Autodesk Inventor part; units mm, degrees
ref_plane "YZ Plane" through (0, 0, 0) normal (1, 0, 0) x (0, 1, 0)
ref_plane "XZ Plane" through (0, 0, 0) normal (0, 1, 0) x (-1, 0, 0)
ref_plane "XY Plane" through (0, 0, 0) normal (0, 0, 1) x (1, 0, 0)
sketch "Szkic1" plane through (0, 0, 0) normal (0, 0, 1) x (1, 0, 0)
  circle A0 centre (0, 0) radius 3
  circle A1 centre (0, 0) radius 6
  point P0 (0, 0)
  dimension "d0" = 12
extrude "Wyciągnięcie proste1" add sketch "Szkic1" against normal blind 1 contours A0 | A1
sketch "Szkic2" plane through (0, 0, 0) normal (0, 0, 1) x (1, 0, 0)
  circle A0 centre (0, 0) radius 6
  circle A1 centre (0, 0) radius 5
  point P0 (0, 0)
  dimension "d3" = 1
extrude "Wyciągnięcie proste2" add sketch "Szkic2" along normal blind 10
full round fillet "Zaokrąglenie1" first side at (4.9353, -0.8021, 6.6667) centre faces at (5.6086, -0.4786, 10) second side at (5.9223, -0.9625, 2.6667)
sketch "Szkic3" plane through (0, 0, 0) normal (0, 1, 0) x (-1, 0, 0)
  line L0 (-6, -1) -> (6, -1)
  line L1 (6, 9.5) -> (-6, 9.5)
  line L2 (0, 3) -> (25, 3)
  line L3 (25, 3) -> (25, -17)
  line L4 (25, -17) -> (0, -17)
  line L5 (0, -17) -> (0, 3)
  line L6 (0, 3) -> (5.5, 3)
  line L7 (5.5, 3) -> (5.5, -1)
  line L8 (5.5, -1) -> (0, -1)
  line L9 (0, -1) -> (0, 3)
  point P0 (0, 0)
  point P1 (5.5, -1)
  point P2 (0, -1)
  dimension "d6" = 25
  dimension "d7" = 20
  dimension "d8" = 5.5
  dimension "d9" = 4
extrude "Wyciągnięcie proste3" add sketch "Szkic3" along normal mid plane 2 contours L0 L7 L2 L3 L4 L5
fillet "Zaokrąglenie2" radius 5 1 edges at (-6, 0, 3)
full round fillet "Zaokrąglenie3" first side at (-20.3316, -0.1112, 3) centre faces at (-25, 0.3333, -10.3333) second side at (-8.3333, -0.3333, -17)
pattern_circular "Szyk kołowy1" count 2 over 360 about axis through (0, 0, 0) along (0, 0, 1) of "Wyciągnięcie proste3", "Zaokrąglenie2", "Zaokrąglenie3"
properties part number "raczka" material "Aluminium 6061"
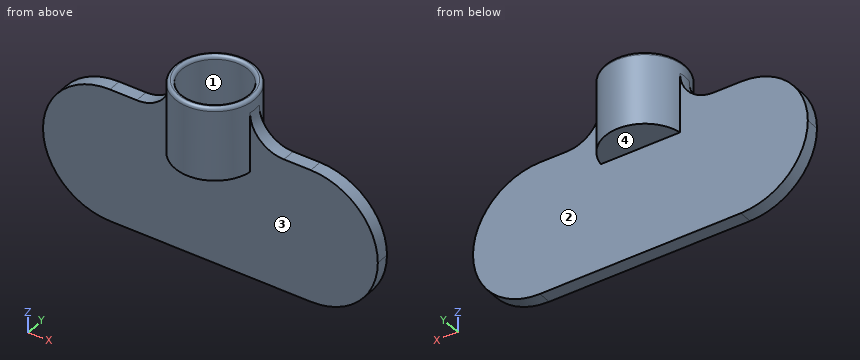
Source: CAD feature listing. Evaluate the final solid. Frame: model axes, mm. Face numbers are marked on the shaded views. Round coordinates to 2 decimals unless told otherwise and drop trailing zeros. Loops run counter-clockwise (first coordinate to the right, second up) from the corner with the lowest first, then second, coordinate; pieces in that order, holes last. Notation, with made-up numbers: M 48,84.25 L 96,84.25 A30 ccw 96,117.25 Z; hole C 55.25,-37.75 d6. An arc over 180 degrees is marked long. Put each result on its own line as item: value.
(1) Ray query, line 1 (Y direction, x = 0, z = 4.5); line 2 (Y direction, x = 9, z = -10.25); line 3 (X direction, y = 2, z = 6.5). Return the intervals inside material, ascending. Write a range as [from, to].
Solutions:
line 1: [-6, -5], [5, 6]
line 2: [-1, 1]
line 3: [-5.66, -4.58], [4.58, 5.66]
(2) First-contact query: pin 1 (3 mm diameter, centred on y = 4.5, z = -2, fed in from +X); pin 2 (8 mm diameter, centred on x = -13.5, z = -8, fed in from -Y); pin 3 (3 mm diameter, centred on x = 0.5, y = 2, fed in from +Z). Flat tips, straight axial feed; report the tip coordinate or a pass-through.
Solutions:
pin 1: x = 4.96
pin 2: y = -1
pin 3: z = 0
(3) Section B-B, the plane z = 8.75. Return loops of the section in (x, y).
Solutions:
outline: C 0,0 d12; hole C 0,0 d10
(4) Pull-direction query (Y, two-part tool) for the marked faces 1, 2, 3 and 4; classes: released by +Y, released by -Y, zero draft, split by the parting line, or undercut.
Solutions:
face 1: undercut
face 2: released by +Y
face 3: released by -Y
face 4: zero draft
(5) Section D-D, the plane z = 4.5. Return loops of the section in (x, y).
Solutions:
outline: M -7.36,-1 L -5.92,-1 A6 ccw 5.92,-1 L 7.36,-1 A7.43 ccw 7.36,1 L 5.92,1 A6 ccw -5.92,1 L -7.36,1 A7.43 ccw Z; hole C 0,0 d10
